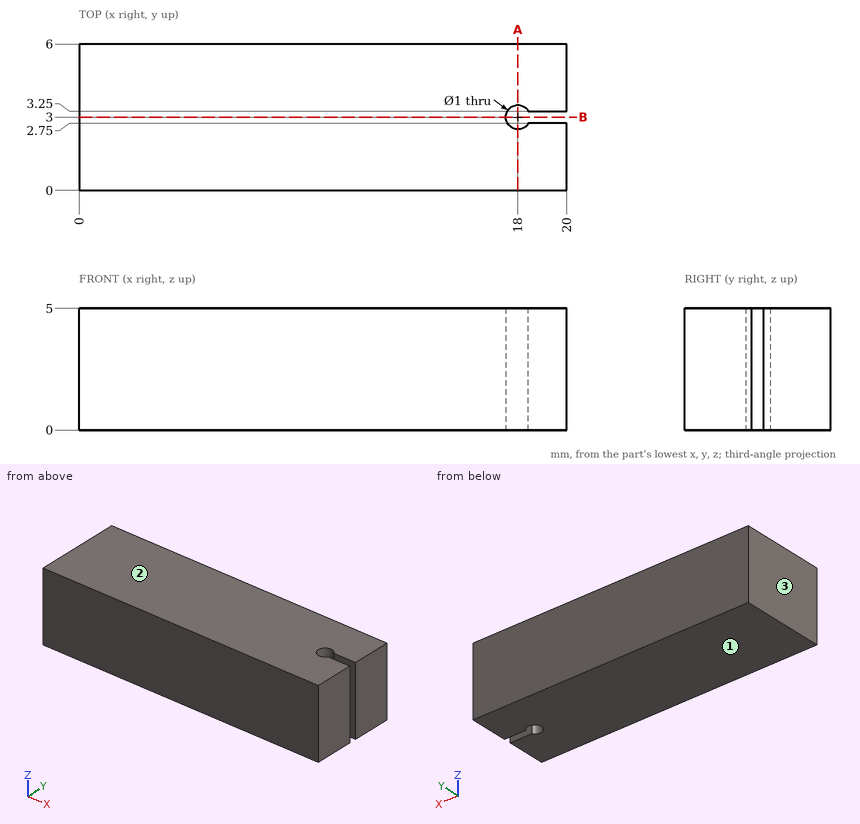
Part print with two shaded views. Sizes in mm from the minimum x, y, z corner. Round coordinates to 2 decimals unless told otherwise and drop trailing zeros. Write each loop counter-clockwise with the first axis right and the second up, starting at its lowest first coordinate (ties: lowest second). Pieces come first, ordered by that corner, then holes. Notation, with made-up numbers: (80, 47.5) -> (94, 47.5) arc R20 cw to (94, 82.5) -> close; hole circle Ø6 at (12, 57). An arc over 180 degrees is marked (long way). Use one line per item in the form item = value.
Q1. Drill centre line: L1, parallel to X at y = 3, z = 2.2. Where is it in solid material? Low to high.
Conclusion:
L1 = 0 to 17.5
Q2. Drop a flat-ended pin along its axis: P1, Ø0.6, axis at x = 18, y = 3, coming from the -Z side. Give the stop position or say it passes through.
Conclusion:
P1 = through
Q3. Two-plate mould, pull along Z, no slides. Class the marked faces 1, 2 and 3: released by +Z, released by -Z, zero draft, split by the parting line, or undercut.
Conclusion:
face_1 = released by -Z
face_2 = released by +Z
face_3 = zero draft
Q4. Band-saw the part on A-A, the plane x = 18. Write the cut outline in (y, z), then the cut area to 3 significant figures.
Conclusion:
outline = (0, 0) -> (2.5, 0) -> (2.5, 5) -> (0, 5) -> close; (3.5, 0) -> (6, 0) -> (6, 5) -> (3.5, 5) -> close
area = 25.0 mm²
Q5. Band-saw the part on B-B, the plane y = 3. Write the cut outline in (x, z).
Conclusion:
outline = (0, 0) -> (17.5, 0) -> (17.5, 5) -> (0, 5) -> close
